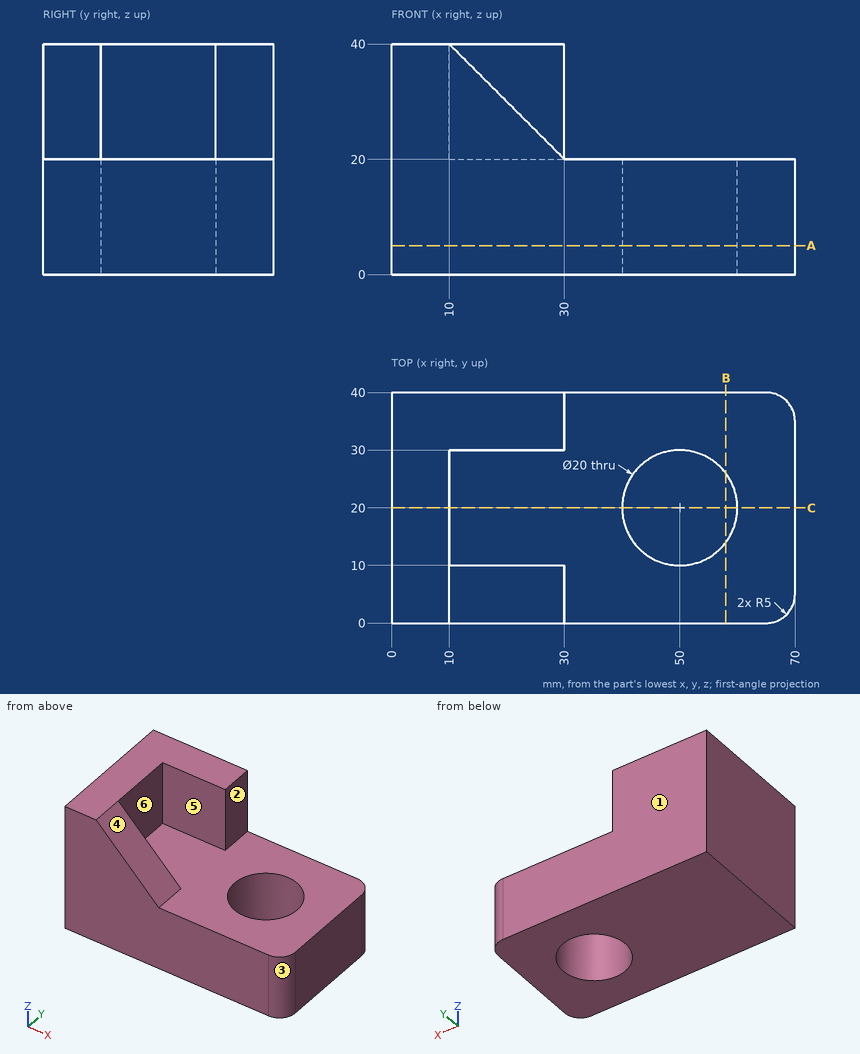
Print and shaded views of the part. All mm, measured from the part's lowest x, y and z. A direction names the side the tool comes from. Coordinates: 2 decimals unless noted, no trailing zeros. Order: outer loops, then holes, each group sorted by start corner. A loop starts at its lowest first (then second) coordinate and runs counter-clockwise, first axis right, second up. Notation, with made-up numbers: (-17.75, 61) -> (-12.75, 61) arc R19 cw to (-12.75, 71) -> close; hole circle Ø8 at (5.25, 49.25). An arc over 180 degrees is marked (long way). Answer as a JSON object with one key per item and string values. Group by question number.
1) Cut at B-B, the plane x = 58. Write the cut outline in (y, z), then the cut area to 3 significant figures.
2) Cut at A-A, the plane z = 5. Write the cut outline in (x, y).
3) Cut at C-C, the plane y = 20. Write the cut outline in (x, z).
4) Pull direction Y, two halves, no side cores. Call the marked faces 3, 4, 5 and 6: +Y half, -Y half, draft (parallel to the pull), parting line (faces both ways), or undercut.
5) Flat gauge pins, fed straight in: pin 1 (12 mm diameter, centred on x = 53, z = 16.5, fed in from -Y); pin 2 (5 mm diameter, centred on y = 37, z = 26, fed in from +X); pin 3 (6 mm diameter, centred on x = 20.5, z = 35, fed in from -Y); pin 4 (1 mm diameter, centred on x = 15.5, y = 15, fed in from +Z). Where does each tip first touch, or does it go through?
6) Drill centre lines: L1, parallel to Y at x = 50, z = 8; L2, parallel to Z at x = 60, y = 29; L3, parallel to Y at x = 51, z = 16. Where is each one in solid material? Low to high.
7) Which spindle directions (+Z, -Z, +X, -X, +Y, -Y) get a long thin tool onto all of the face, cutting with end or side? Do the marked faces 1 and 2. Say none if no direction does.
Check values:
{
 "1": {"outline": "(0, 0) -> (14, 0) -> (14, 20) -> (0, 20) -> close; (26, 0) -> (40, 0) -> (40, 20) -> (26, 20) -> close", "area": "560 mm²"},
 "2": {"outline": "(0, 0) -> (65, 0) arc R5 ccw to (70, 5) -> (70, 35) arc R5 ccw to (65, 40) -> (0, 40) -> close; hole circle Ø20 at (50, 20)"},
 "3": {"outline": "(0, 0) -> (40, 0) -> (40, 20) -> (10, 20) -> (10, 40) -> (0, 40) -> close; (60, 0) -> (70, 0) -> (70, 20) -> (60, 20) -> close"},
 "4": {"face 3": "-Y half", "face 4": "draft", "face 5": "undercut", "face 6": "undercut"},
 "5": {"pin 1": "stops at y = 0", "pin 2": "stops at x = 30", "pin 3": "stops at y = 30", "pin 4": "stops at z = 20"},
 "6": {"L1": "y = 0 to 10, 30 to 40", "L2": "z = 0 to 20", "L3": "y = 0 to 10.05, 29.95 to 40"},
 "7": {"face 1": "+Z, -Z, +X, -X, +Y", "face 2": "+Z, +X, +Y, -Y"}
}
